Source: CAD feature listing. Evaluate the final solid. Frame: model axes, mm. A direction names the side the tool comes from. Give positions to 0.01 mm unless a question says otherwise; leave off trailing zeros. Write each loop counter-clockwise with the first axis right and the second up, starting at its lowest first coordinate (ties: lowest second). Pieces come first, ordered by that corner, then holes. Notation, with made-up numbers: M -3.75,84.25 L 49.25,84.25 A12 cw 49.25,93.25 Z; hole C -20,17 d10. An arc over 180 degrees is marked long. Use CSV: the item, a comma, the result in double quotes. Start each with the question number.
from build123d import *

# Parameters (mm, degrees)
SKETCH1_R           = 6
SKETCH1_R_2         = 4
BOSS_EXTRUDE1_DEPTH = 3.5
SKETCH2_R           = 5.75
SKETCH2_R_2         = 4.25
CUT_EXTRUDE1_DEPTH  = 0.2
CUT_EXTRUDE2_START  = -3.5
SKETCH2_2_R         = 5.75
SKETCH2_2_R_2       = 4.25
CUT_EXTRUDE2_DEPTH  = 0.2


with BuildPart() as part:
    # Sketch1 → Boss-Extrude1 (new body)
    with BuildSketch(Plane(origin=(0, 0, 0), x_dir=(1, 0, 0), z_dir=(0, 1, 0))):
        Circle(SKETCH1_R)
        Circle(SKETCH1_R_2, mode=Mode.SUBTRACT)
    extrude(amount=BOSS_EXTRUDE1_DEPTH)

    # Sketch2 → Cut-Extrude1 (cut)
    with BuildSketch(Plane(origin=(0, 3.5, 0), x_dir=(1, 0, 0), z_dir=(0, 1, 0))):
        Circle(SKETCH2_R)
        Circle(SKETCH2_R_2, mode=Mode.SUBTRACT)
    extrude(amount=-CUT_EXTRUDE1_DEPTH, mode=Mode.SUBTRACT)

    # Sketch2<2> → Cut-Extrude2 (cut)
    with BuildSketch(Plane(origin=(0, 3.5, 0), x_dir=(1, 0, 0), z_dir=(0, 1, 0)).offset(CUT_EXTRUDE2_START)):
        Circle(SKETCH2_2_R)
        Circle(SKETCH2_2_R_2, mode=Mode.SUBTRACT)
    extrude(amount=CUT_EXTRUDE2_DEPTH, mode=Mode.SUBTRACT)


solid = part.part
Item 1: Contact query for flat-ended pins moving along their axis: pin 1 Ø3.5 at (x, z) = (0.5, 2) entering from +Y (3 decimals); pin 2 Ø6 at (x, z) = (-2.5, -1) entering from +Y; pin 3 Ø2 at (x, y) = (-2, 1) entering from -Z. Output: stop coordinate, or through.
Item 2: Set-up query: faces 1 (the cylindrical face through (-0.867, 1.726, 3.905)), 2 (the flat face through (-2, 3.3, 4)). Return all of +Z, -Z, +X, -X, +Y, -Y with unobstructed straight access to the full face (end or side cutting, diameter ignored); none if empty.
Item 3: Pull-direction query (X, two-part tool) for faces 3 (the cylindrical face through (-6, 2, 0)), 4 (the flat face through (-2, 0.2, 4)); classes: released by +X, released by -X, zero draft, split by the parting line, or undercut.
Item 4: Section C-C (y = 2.55). Return the cut outline in (x, z).
Item 5: Section B-B (x = 0). Return the cut outline in (y, z), plus the area to 3 significant figures.
Item 6: Material intervals for probe 1 along X at (y, z) = (0.15, 0); probe 2 along Z at (x, y) = (0, 2.6), sorted ascending.
Item 7: Section A-A (z = 0). Return the cut outline in (x, y), plus the area to 3 significant figures.
Item 8: Section D-D (x = 4.5). Return the cut outline in (y, z), plus the area to 3 significant figures.
Output values:
1,pin 1,"passes through"
1,pin 2,"stops at y = 3.5"
1,pin 3,"stops at z = -5.92"
2,face 1,"+Y, -Y"
2,face 2,"+Y"
3,face 3,"split by the parting line"
3,face 4,"undercut"
4,outline,"C 0,0 d12; hole C 0,0 d8"
5,outline,"M 0,-6 L 3.5,-6 L 3.5,-5.75 L 3.3,-5.75 L 3.3,-4.25 L 3.5,-4.25 L 3.5,-4 L 0,-4 L 0,-4.25 L 0.2,-4.25 L 0.2,-5.75 L 0,-5.75 Z; M 0,4 L 3.5,4 L 3.5,4.25 L 3.3,4.25 L 3.3,5.75 L 3.5,5.75 L 3.5,6 L 0,6 L 0,5.75 L 0.2,5.75 L 0.2,4.25 L 0,4.25 Z"
5,area,"12.8 mm2"
6,probe 1,"x = -6 to -5.75, -4.25 to -4, 4 to 4.25, 5.75 to 6"
6,probe 2,"z = -6 to -4, 4 to 6"
7,outline,"M -6,0 L -5.75,0 L -5.75,0.2 L -4.25,0.2 L -4.25,0 L -4,0 L -4,3.5 L -4.25,3.5 L -4.25,3.3 L -5.75,3.3 L -5.75,3.5 L -6,3.5 Z; M 4,0 L 4.25,0 L 4.25,0.2 L 5.75,0.2 L 5.75,0 L 6,0 L 6,3.5 L 5.75,3.5 L 5.75,3.3 L 4.25,3.3 L 4.25,3.5 L 4,3.5 Z"
7,area,"12.8 mm2"
8,outline,"M 0,-3.97 L 3.5,-3.97 L 3.5,-3.58 L 3.3,-3.58 L 3.3,3.58 L 3.5,3.58 L 3.5,3.97 L 0,3.97 L 0,3.58 L 0.2,3.58 L 0.2,-3.58 L 0,-3.58 Z"
8,area,"24.9 mm2"
